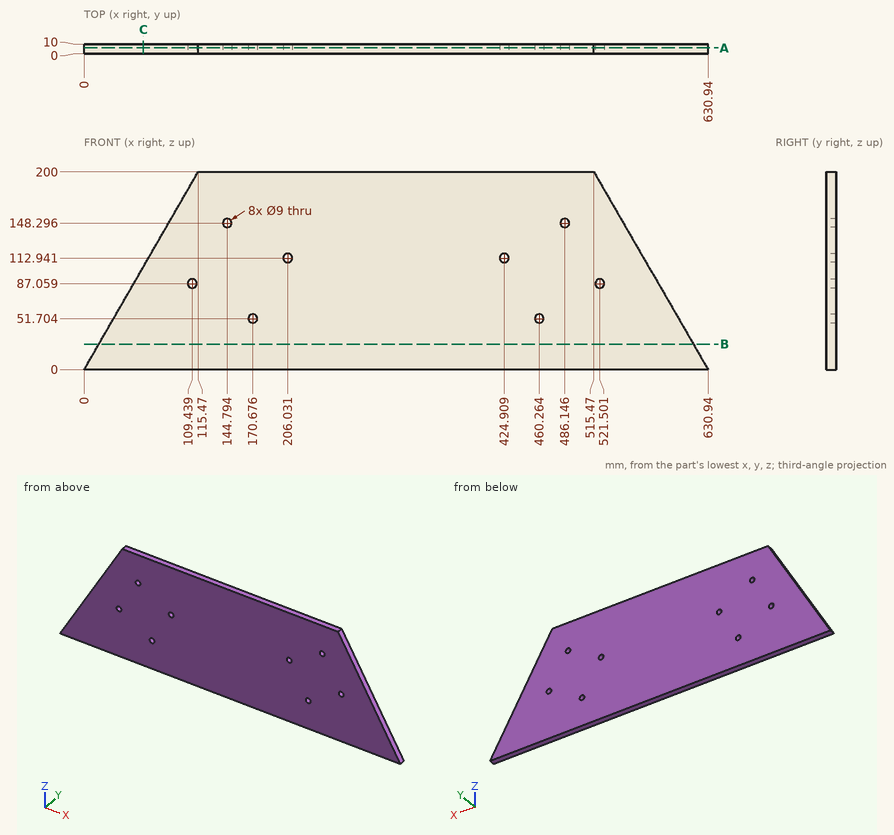
Drawing for the job (mm, zero at the part's lowest x, y, z). Round coordinates to 2 decimals unless told otherwise and drop trailing zeros. Write each loop counter-clockwise with the first axis right and the second up, starting at its lowest first coordinate (ties: lowest second). Pieces come first, ordered by that corner, then holes. Notation, with made-up numbers: M 0,9.25 L 53,9.25 A10 cw 53,15.25 Z; hole C 33,74.25 d5. An arc over 180 degrees is marked long. One line per question, with ' | ' between items.
1. Pin check, flat tips, straight feed: pin 1 Ø6 at (y, z) = (3.5, 41.5) entering from +X; pin 2 Ø1 at (y, z) = (6.5, 99) entering from -X; pin 3 Ø1 at (x, y) = (105, 7) entering from +Z. Stop position of each tip, or through.
Working result:
pin 1: x = 608.71 | pin 2: x = 56.87 | pin 3: z = 182.73
2. Cut at B-B on z = 26. Write the cut outline in (x, y), and give its area (3 significant figures).
Working result:
outline: M 15.01,0 L 615.93,0 L 615.93,10 L 15.01,10 Z | area: 6,010 mm2
3. Cut at C-C on x = 60. Write the cut outline in (y, z).
Working result:
outline: M 0,0 L 10,0 L 10,103.92 L 0,103.92 Z
4. Probe L1, parallel to X at y = 0.75, z = 149.5 (1 decimal); L2, parallel to X at y = 7, z = 90.5; L3, parallel to Z at x = 208, y = 1.5 (1 decimal). List the from-to ranges inside material, lowest first. Write a range as from..to.
Working result:
L1: 86.3..140.5, 149.1..481.8, 490.5..544.6 | L2: 52.25..106.54, 112.34..518.6, 524.4..578.69 | L3: 0..108.9, 117..200
5. Cut at A-A on y = 6. Count the separate pieces of the cut face and the enclosed holes in it, and give its area (3 significant figures).
Working result:
separate pieces: 1 | enclosed holes: 8 | area: 103,000 mm2
